from build123d import *

# Parameters (mm, degrees)
F1_R = 10


with BuildPart() as f2:
    # F2: sweep along a path in F0
    with BuildLine(Plane.XY) as f2_path:
        Line((0, 0), (70, 0))
        ThreePointArc((70, 0), (91.2132034356, 8.7867965644), (100, 30))
        Line((100, 30), (100, 70))
        ThreePointArc((100, 70), (108.7867965644, 91.2132034356), (130, 100))
        Line((130, 100), (200, 100))
    # F1 (on Right) → F2 (sweep)
    with BuildSketch(Plane.YZ):
        Circle(F1_R)
    sweep(path=f2_path.line)


solid = f2.part
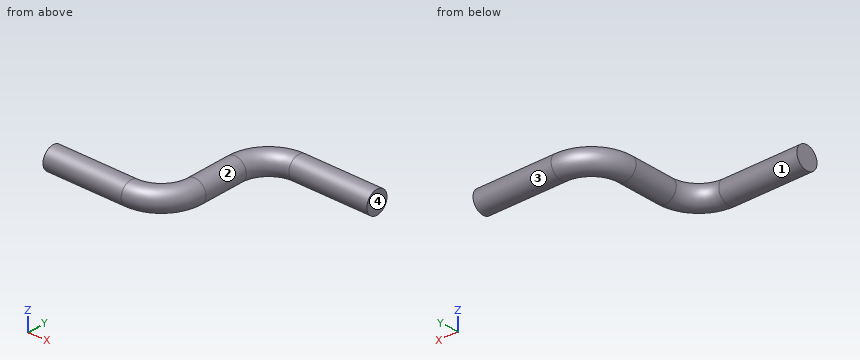
Geometry check sheet. Reference: the model listing, model coordinates, mm. Face numbers are marked on the shaded views. A direction names the side the tool comes from. Round coordinates to 2 decimals unless told otherwise and drop trailing zeros. Loops run counter-clockwise (first coordinate to the right, second up) from the corner with the lowest first, then second, coordinate; pieces in that order, holes last. Notation, with made-up numbers: (59.25, -21) - (70.25, -21) arc R19 cw to (70.25, 7) - close; hole circle Ø4 at (58.25, 86). An arc over 180 degrees is marked (long way). One line per question, with ' | ' between items. Start each with the question number.
1. Scan lines: line 1 (Y direction, x = 32, z = -1.75); line 2 (Y direction, x = 38, z = -0.5); line 3 (X direction, y = 43.5, z = -2). Record each from-to range of solid material in increasing order. Write a range as [from, to].
2. Depth check by flat-ended pin: pin 1 (3 mm diameter, centred on y = 65, z = 5.5, fed in from +X); pin 2 (5 mm diameter, centred on y = 19.5, z = 2, fed in from -X); pin 3 (8 mm diameter, centred on x = 176, z = -6, fed in from -Y). Enter the tip coordinate at first touch or a pass-through.
3. Cross-section at B-B on x = 16.5. Record the cut outline in (y, z).
4. Cross-section at C-C on y = 60. Record the cut outline in (x, z).
5. Tool access check on the marked faces 1, 2, 3 and 4. Record the directions out of +Z, -Z, +X, -X, +Y, -Y that give a thin tool (end or side, any length) a straight path to the whole face; none if there is none.
6. Cross-section at A-A on z = -8. Record the cut outline in (x, y).
Taken from the geometry:
1) line 1: [-9.85, 9.85] | line 2: [-9.99, 9.99] | line 3: [90.2, 109.8]
2) pin 1: x = 109.17 | pin 2: x = 85.39 | pin 3: y = 90.2
3) outline: circle Ø20 at (0, 0)
4) outline: circle Ø20 at (100, 0)
5) face 1: -X | face 2: none | face 3: +X | face 4: +Z, -Z, +X, +Y, -Y
6) outline: (0, -6) - (70, -6) arc R36 ccw to (106, 30) - (106, 70) arc R24 cw to (130, 94) - (200, 94) - (200, 106) - (130, 106) arc R36 ccw to (94, 70) - (94, 30) arc R24 cw to (70, 6) - (0, 6) - close
